Geometry check sheet. Reference: the model listing, model coordinates, mm. A direction names the side the tool comes from. Round coordinates to 2 decimals unless told otherwise and drop trailing zeros. Write each loop counter-clockwise with the first axis right and the second up, starting at its lowest first coordinate (ties: lowest second). Pieces come first, ordered by that corner, then holes.
from build123d import *

# Parameters (mm, degrees)
BOSS_EXTRUDE1_DEPTH = 1.524


with BuildPart() as part:
    # Sketch1 → Boss-Extrude1 (new body)
    with BuildSketch(Plane.XY):
        Polygon((-9.60258928, -1.524), (-28.761615364, -5.146272329), (-28.478498191, -6.643743753), (-31.47344104, -7.209978099), (-31.756558213, -5.712506675), (-40.495294208, -7.364682597), (-40.212177035, -8.862154021), (-43.207119883, -9.428388367), (-43.490237056, -7.930916943), (-48.355985293, -8.850852284), (-53.593355447, -8.096704042), (-53.810561584, -9.605146117), (-56.827445734, -9.170733844), (-56.610239597, -7.662291769), (-78.191926721, -4.554665056), (-78.409132858, -6.063107132), (-81.426017008, -5.628694858), (-81.208810872, -4.120252783), (-99.239134473, -1.524), (-68.783094529, -1.524), (-68.783094529, 0), (-63.703094529, 0), (-63.703094529, -1.524), (-39.202780194, -1.524), (-39.202780194, 0), (-34.122780194, 0), (-34.122780194, -1.524), align=None)
    extrude(amount=-BOSS_EXTRUDE1_DEPTH)


solid = part.part
1. Section check C-C (x = -25). Record the cut outline in (y, z).
2. Scan lines: line 1 along X through (y, z) = (-0.75, -1.1); line 2 along Y through (x, z) = (-60, -0.7); line 3 along Y through (x, z) = (-44.5, -0.85). Record each from-to range of solid material in increasing order.
3. Access from +Z, -Z, +X, -X, +Y, -Y to the whole of each face (thin tool, end or side, straight path). Record for faces 1 (the face through (-53.7, -8.84, -0.75)), 2 (the face through (-34.123, -1, -1)), 3 (the face through (-68.783, -1, -1)), 4 (the face through (-63.703, -1, -1)), 5 (the face through (-28.622, -5.885, -0.751)).
4. Section check A-A (z = -1). Record the cut outline in (x, y).
5. Section check B-B (y = -2.5). Record the cut outline in (x, z).
6. Depth check by flat-ended pin: pin 1 Ø0.5 at (x, z) = (-50.5, -1) entering from +Y; pin 2 Ø0.8 at (y, z) = (-0.5, -0.5) entering from +X; pin 3 Ø0.8 at (y, z) = (-0.5, -1) entering from -X. Enter the tip coordinate at first touch or a pass-through.
7. Release check for a two-part mould opening along X. For faces 6 (the face through (-40.356, -8.103, -0.751)), 7 (the face through (-50.94, -8.48, -0.75)), 8 (the face through (-37, 0, -1)) record: +X half, -X half, draft (parallel to the pull), parting line (faces both ways), or undercut.
Results below:
1. outline: (-4.44, -1.52) - (-1.52, -1.52) - (-1.52, 0) - (-4.44, 0) - close
2. line 1: x = -68.78 to -63.7, -39.2 to -34.12
2. line 2: y = -7.17 to -1.52
2. line 3: y = -8.12 to -1.52
3. face 1: +Z, -Z, -Y
3. face 2: +Z, -Z, +X, +Y
3. face 3: +Z, -Z, -X, +Y
3. face 4: +Z, -Z, +Y
3. face 5: +Z, -Z, +X
4. outline: (-99.24, -1.52) - (-81.21, -4.12) - (-81.43, -5.63) - (-78.41, -6.06) - (-78.19, -4.55) - (-56.61, -7.66) - (-56.83, -9.17) - (-53.81, -9.61) - (-53.59, -8.1) - (-48.36, -8.85) - (-43.49, -7.93) - (-43.21, -9.43) - (-40.21, -8.86) - (-40.5, -7.36) - (-31.76, -5.71) - (-31.47, -7.21) - (-28.48, -6.64) - (-28.76, -5.15) - (-9.6, -1.52) - (-34.12, -1.52) - (-34.12, 0) - (-39.2, 0) - (-39.2, -1.52) - (-63.7, -1.52) - (-63.7, 0) - (-68.78, 0) - (-68.78, -1.52) - close
5. outline: (-92.46, -1.52) - (-14.76, -1.52) - (-14.76, 0) - (-92.46, 0) - close
6. pin 1: stops at y = -1.52
6. pin 2: stops at x = -34.12
6. pin 3: stops at x = -68.78
7. face 6: +X half
7. face 7: undercut
7. face 8: draft
